Autodesk Inventor part; units mm, degrees
ref_plane "YZ Plane" through (0, 0, 0) normal (1, 0, 0) x (0, 1, 0)
ref_plane "XZ Plane" through (0, 0, 0) normal (0, 1, 0) x (-1, 0, 0)
ref_plane "XY Plane" through (0, 0, 0) normal (0, 0, 1) x (1, 0, 0)
sketch "Esquisse1" plane through (0, 0, 0) normal (0, 0, 1) x (1, 0, 0)
  line L0 (-29, 24.5) -> (29, 24.5) construction
  line L1 (29, 24.5) -> (29, -24.5) construction
  line L2 (29, -24.5) -> (-29, -24.5) construction
  line L3 (-29, -24.5) -> (-29, 24.5) construction
  line L4 (-29, 24.5) -> (29, -24.5) construction
  line L5 (29, 24.5) -> (-29, -24.5) construction
  circle A0 centre (29, 24.5) radius 1.65
  circle A1 centre (-29, 24.5) radius 1.65
  circle A2 centre (-29, -24.5) radius 1.65
  circle A3 centre (29, -24.5) radius 1.65
  circle A4 centre (29, 24.5) radius 3
  circle A5 centre (-29, 24.5) radius 3
  circle A6 centre (-29, -24.5) radius 3
  circle A7 centre (29, -24.5) radius 3
  line L6 (-42, -27.5) -> (-32, -27.5)
  line L7 (-32, -27.5) -> (-32, 27.5)
  line L8 (-32, 27.5) -> (-42, 27.5)
  line L9 (-42, 27.5) -> (-42, -27.5)
  line L10 (-42, -27.5) -> (-32, 27.5) construction
  line L11 (-32, -27.5) -> (-42, 27.5) construction
  line L12 (-50, -27.5) -> (-42, -27.5)
  line L13 (-42, -27.5) -> (-42, 27.5)
  line L14 (-42, 27.5) -> (-50, 27.5)
  line L15 (-50, 27.5) -> (-50, -27.5)
  line L16 (-50, -27.5) -> (-42, 27.5) construction
  line L17 (-42, -27.5) -> (-50, 27.5) construction
  line L18 (-74.4, 0) -> (96.4, 0)
  line L19 (-32, -27.5) -> (32, -27.5)
  line L20 (32, -27.5) -> (32, 27.5)
  line L21 (32, 27.5) -> (-32, 27.5)
  line L22 (-32, 27.5) -> (-32, -27.5)
  line L23 (-32, -27.5) -> (32, 27.5) construction
  line L24 (32, -27.5) -> (-32, 27.5) construction
  line L25 (26.8787, 22.3787) -> (-26.8787, 22.3787)
  line L26 (-26.8787, 22.3787) -> (-26.8787, -22.3787)
  line L27 (-26.8787, -22.3787) -> (26.8787, -22.3787)
  line L28 (26.8787, -22.3787) -> (26.8787, 22.3787)
  line L29 (26.8787, 22.3787) -> (-26.8787, -22.3787) construction
  line L30 (-26.8787, 22.3787) -> (26.8787, -22.3787) construction
  line L31 (26.8787, 0) -> (32, 0) construction
  line L32 (0, -22.3787) -> (0, -27.5) construction
  line L33 (72, -3.5) -> (32, -3.5)
  line L34 (32, -3.5) -> (32, 3.5)
  line L35 (32, 3.5) -> (72, 3.5)
  line L36 (72, 3.5) -> (72, -3.5)
  line L37 (72, -3.5) -> (32, 3.5) construction
  line L38 (32, -3.5) -> (72, 3.5) construction
  circle A8 centre (68.5, 0) radius 3.5
  circle A9 centre (68.5, 0) radius 1.65
  point P0 (0, 0)
  point P1 (-29, 0)
  point P2 (0, -24.5)
  point P3 (-37, 0)
  point P4 (-46, 0)
  point P5 (-32, 0)
  point P6 (-29, -27.5)
  point P7 (29, -27.5)
  point P8 (32, -24.5)
  point P9 (-29, 27.5)
  point P10 (-32, 24.5)
  point P11 (-32, -24.5)
  point P12 (32, 24.5)
  point P13 (29, 27.5)
  point P14 (52, 0)
  point P15 (68.5, -3.5)
  point P16 (68.5, 3.5)
  dimension "d3" = 6
  dimension "d0" = 49
  dimension "d1" = 58
  dimension "d2" = 3.3
  dimension "d32" = 10
  dimension "d33" = 8
  dimension "d49" = 7
  dimension "d50" = 40
extrude "Extrusion1" add sketch "Esquisse1" against normal blind 4 contours A4 | L25 A5 L21 A4 | A4 L20 L18 L28 | A5 | L26 L18 L7 A5 | L18 L20 A7 L28 | L35 A8 L18 L20 | A5 L7 L21 | L7 L18 L9 L8 | L26 A6 L7 L18 | L18 A8 L33 L20 | A7 | A7 L19 A6 L27 | A8 L18 A9 | L7 L6 L9 L18 | A6 | L18 A9 A8 | L9 L18 L15 L14 | A6 L19 L7 | L9 L12 L15 L18
extrude "Extrusion10" add sketch "Esquisse1" along normal blind 12 contours L9 L18 L15 L14 | L9 L12 L15 L18
extrude "Extrusion11" add sketch "Esquisse1" along normal blind 6 contours A4 | A5 | A7 | A8 L18 A9 | A6 | L18 A9 A8
sketch "Esquisse13" plane through (-42, -27.5, 0) normal (1, 0, 0) x (0, 0, -1)
  line L0 (0, 55) -> (0, 0)
  line L1 (0, 55) -> (-12, 55)
  line L2 (-12, 0) -> (-12, 55)
  line L3 (0, 0) -> (-12, 0)
  line L4 (0, 0) -> (-12, 0)
  line L5 (-6, 0) -> (-6, 12.5)
  line L6 (-6, 12.5) -> (-6, 42.5) construction
  line L7 (-6, 42.5) -> (-6, 55)
  line L8 (0, 55) -> (-12, 55)
  circle A0 centre (-6, 12.5) radius 2.1
  circle A1 centre (-6, 42.5) radius 2.1
  line L9 (-2, 14.8094) -> (-2, 10.1906)
  line L10 (-2, 10.1906) -> (-6, 7.8812)
  line L11 (-6, 7.8812) -> (-10, 10.1906)
  line L12 (-10, 10.1906) -> (-10, 14.8094)
  line L13 (-10, 14.8094) -> (-6, 17.1188)
  line L14 (-6, 17.1188) -> (-2, 14.8094)
  line L15 (-6, 37.8812) -> (-10, 40.1906)
  line L16 (-10, 40.1906) -> (-10, 44.8094)
  line L17 (-10, 44.8094) -> (-6, 47.1188)
  line L18 (-6, 47.1188) -> (-2, 44.8094)
  line L19 (-2, 44.8094) -> (-2, 40.1906)
  line L20 (-2, 40.1906) -> (-6, 37.8812)
  point P0 (-10, 42.5)
  dimension "d38" = 4.2
  dimension "d39" = 8
  dimension "d41" = 30
extrude "Extrusion12" cut sketch "Esquisse13" against normal through all contours A1 | A0
extrude "Extrusion13" cut sketch "Esquisse13" against normal blind 4 contours L18 L19 L20 L15 L16 L17 | L11 L12 L13 L14 L9 L10
chamfer "Chanfrein2" distance 0.5 angle 45 4 edges at (-32, -24.5, 6) (26, -24.5, 6) (26, 24.5, 6) (-32, 24.5, 6)
properties part number "Support_Raspberry"
Model file for the job. Use its own axes, mm. A direction names the side the tool comes from. Coordinates: 2 decimals unless noted, no trailing zeros. Order: outer loops, then holes, each group sorted by start corner. A loop starts at its lowest first (then second) coordinate and runs counter-clockwise, first axis right, second up. Notation, with made-up numbers: (30, 85.25) - (60, 85.25) arc R22 cw to (60, 109.25) - close; hole circle Ø1 at (-1, -22). An arc over 180 degrees is marked (long way). Return JSON: item names as keys, results as strings. Group by question number.
1) Saw through at B-B, the plane y = 15. Write the cut outline in (x, z), plus the area to 3 significant figures.
2) Mould opens along X. For faces 6 (the flat face through (32, 14, -2)), 7 (the flat face through (-26.879, 0, -2)), 8 (the flat face through (51, -3.5, -2)) say: released by +X, released by -X, zero draft, split by the parting line, or undercut.
3) Tool access for faces 1 (the cylindrical face through (-47.97, 16.77, 4.87)), 2 (the flat face through (-35, 0, 0)), 3 (the flat face through (-43.972, -18.448, 3.972)), 4 (the flat face through (70, -1, 6)), 5 (the flat face through (0, -22.379, -2)): list every direction of +Z, -Z, +X, -X, +Y, -Y with a clear straight run to the whole face (end or side of a thin tool).
4) Saw through at C-C, the plane z = -2. Write the cut outline in (x, y).
5) Saw through at A-A, the plane x = 11. Write the cut outline in (y, z).
6) Saw through at D-D, the plane y = -11.5. Write the cut outline in (x, z).
7) Flat gauge pins, fed straight in: P1, Ø4, axis at x = 28, y = -25, coming from the +Z side; P2, Ø6, axis at y = -12, z = 10, coming from the +X side; P3, Ø4.5, axis at y = -10.5, z = -2.5, coming from the +X side. Where does each tip first touch, or does it go through?
8) Probe line 1 (Y direction, x = -49.2, z = 6); line 2 (Y direction, x = 29, z = -0.75); line 3 (X direction, y = 0, z = 2). List the from-to ranges inside material, lowest first. Write a range as from..to.
Values found:
{
 "1": {"outline": "(-50, -4) - (-26.88, -4) - (-26.88, 0) - (-42, 0) - (-42, 2) - (-46, 2) - (-46, 3.9) - (-50, 3.9) - close; (-50, 8.1) - (-46, 8.1) - (-46, 10) - (-42, 10) - (-42, 12) - (-50, 12) - close; (26.88, -4) - (32, -4) - (32, 0) - (26.88, 0) - close", "area": "160 mm²"},
 "2": {"face 6": "released by +X", "face 7": "undercut", "face 8": "zero draft"},
 "3": {"face 1": "+X, -X", "face 2": "+Z", "face 3": "+X", "face 4": "+Z, +X, +Y, -Y", "face 5": "+Z, -Z"},
 "4": {"outline": "(-50, -27.5) - (29, -27.5) arc R3 ccw to (32, -24.5) - (32, -3.5) - (68.5, -3.5) arc R3.5 ccw to (68.5, 3.5) - (32, 3.5) - (32, 24.5) arc R3 ccw to (29, 27.5) - (-50, 27.5) - close; hole circle Ø3.3 at (-29, -24.5); hole circle Ø3.3 at (-29, 24.5); hole (-26.88, -22.38) - (26.88, -22.38) - (26.88, 22.38) - (-26.88, 22.38) - close; hole circle Ø3.3 at (29, -24.5); hole circle Ø3.3 at (29, 24.5); hole circle Ø3.3 at (68.5, 0)"},
 "5": {"outline": "(-27.5, -4) - (-22.38, -4) - (-22.38, 0) - (-27.5, 0) - close; (22.38, -4) - (27.5, -4) - (27.5, 0) - (22.38, 0) - close"},
 "6": {"outline": "(-50, -4) - (-26.88, -4) - (-26.88, 0) - (-42, 0) - (-42, 4.06) - (-46, 4.06) - (-46, 7.94) - (-42, 7.94) - (-42, 12) - (-50, 12) - close; (26.88, -4) - (32, -4) - (32, 0) - (26.88, 0) - close"},
 "7": {"P1": "stops at z = 6", "P2": "stops at x = -42", "P3": "stops at x = 32"},
 "8": {"line 1": "y = -27.5..-17.1, -12.9..12.9, 17.1..27.5", "line 2": "y = -27.5..-26.15, -22.85..22.85, 26.15..27.5", "line 3": "x = -50..-42, 65..66.85, 70.15..72"}
}
